```python
from build123d import *

# Parameters (mm, degrees)
SKETCH1_W                       = 44
SKETCH1_H                       = 150
BOSS_EXTRUDE1_DEPTH             = 8
CUT_EXTRUDE3_DEPTH              = 5
SKETCH3_OUTSIDE_W               = 77.304
SKETCH3_OUTSIDE_H               = 183.304
CUT_EXTRUDE4_DEPTH              = 8
CBORE_FOR_M3_SBHCS1_D           = 3.4
CBORE_FOR_M3_SBHCS1_CBORE_D     = 6.7
CBORE_FOR_M3_SBHCS1_CBORE_DEPTH = 1.65


with BuildPart() as part:
    # Sketch1 → Boss-Extrude1 (new body)
    with BuildSketch(Plane(origin=(0, 0, 0), x_dir=(0, 0, -1), z_dir=(1, 0, 0))):
        with Locations((22, 75)):
            Rectangle(SKETCH1_W, SKETCH1_H)
    extrude(amount=BOSS_EXTRUDE1_DEPTH)

    # Sketch2 → Cut-Extrude3 (cut)
    with BuildSketch(Plane(origin=(0, 0, 0), x_dir=(0, 0, -1), z_dir=(1, 0, 0))):
        Polygon((22, 19), (18.535898385, 17), (18.535898385, 13), (22, 11), (25.464101615, 13), (25.464101615, 17), align=None)
    extrude(amount=CUT_EXTRUDE3_DEPTH, mode=Mode.SUBTRACT)

    # Sketch3 outside → Cut-Extrude4 (cut)
    with BuildSketch(Plane(origin=(8, 0, 0), x_dir=(0, 0, -1), z_dir=(1, 0, 0))):
        with Locations((22, 75)):
            Rectangle(SKETCH3_OUTSIDE_W, SKETCH3_OUTSIDE_H)
        with BuildLine():
            Line((11, 150), (11, 28.564659966))
            ThreePointArc((11, 28.564659966), (10.591663047, 25.736232842), (9.4, 23.13879598))
            ThreePointArc((9.4, 23.13879598), (22, 0), (34.6, 23.13879598))
            ThreePointArc((34.6, 23.13879598), (33.408336953, 25.736232842), (33, 28.564659966))
            Line((33, 28.564659966), (33, 150))
            Line((33, 150), (11, 150))
        make_face(mode=Mode.SUBTRACT)
    extrude(amount=-CUT_EXTRUDE4_DEPTH, mode=Mode.SUBTRACT)

    # CBORE for M3 SBHCS1 (through all)
    with Locations(Plane(origin=(8, 0, 0), x_dir=(0, 0, -1), z_dir=(1, 0, 0))):
        with Locations((22, 15)):
            CounterBoreHole(CBORE_FOR_M3_SBHCS1_D / 2, CBORE_FOR_M3_SBHCS1_CBORE_D / 2, CBORE_FOR_M3_SBHCS1_CBORE_DEPTH)


solid = part.part
```
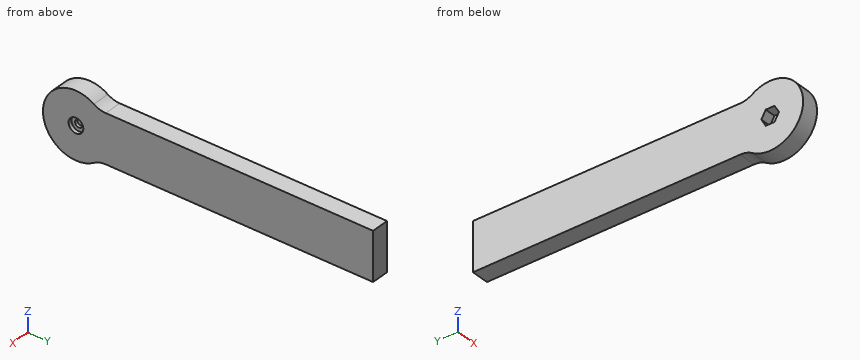
CAD build for the part. Positions are in the model's coordinates, mm. Give positions to 0.01 mm unless a question says otherwise; leave off trailing zeros. Write each loop counter-clockwise with the first axis right and the second up, starting at its lowest first coordinate (ties: lowest second). Pieces come first, ordered by that corner, then holes. Notation, with made-up numbers: M 40,12 L 73,12 A34 ccw 73,43 Z; hole C 60,78 d6. An arc over 180 degrees is marked long. Return JSON: item names as keys, results as strings. Group by question number.
(1) Flat gauge pins, fed straight in: pin 1 Ø1 at (x, y) = (1.5, 108) entering from -Z; pin 2 Ø4 at (x, y) = (5, 122) entering from +Z; pin 3 Ø2 at (y, z) = (14, -22.5) entering from -X. Where does each tip first touch, or does it go through?
(2) Band-saw the part on A-A (y = 15). Give the cut face in (x, z), and give its area (3 significant figures).
(3) Band-saw the part on B-B (x = 1.75). Give the cut face in (y, z), and give its area (3 significant figures).
(4) Band-saw the part on C-C (y = 98). Give the cut face in (x, z), and give its area (3 significant figures).
(5) Band-saw the part on D-D (z = -13.5). Give the cut face in (x, y), and give its area (3 significant figures).
(6) Drill centre lines: L1, parallel to Y at x = 7.05, z = -22; L2, parallel to Y at x = 5.5, z = -22; L3, parallel to Z at x = 4.75, y = 40. Where is each one in solid material? Low to high. Write a range as [from, to].
Entries:
{
 "1": {"pin 1": "stops at z = -33", "pin 2": "stops at z = -11", "pin 3": "stops at x = 5"},
 "2": {"outline": "M 0,-37 L 8,-37 L 8,-25.35 L 6.35,-25.35 L 6.35,-23.7 L 5,-23.7 L 5,-25.46 L 0,-25.46 Z; M 0,-18.54 L 5,-18.54 L 5,-20.3 L 6.35,-20.3 L 6.35,-18.65 L 8,-18.65 L 8,-7 L 0,-7 Z", "area": "190 mm^2"},
 "3": {"outline": "M 23.14,-34.6 A10 cw 28.56,-33 L 150,-33 L 150,-11 L 28.56,-11 A10 cw 23.14,-9.4 A15 ccw long Z; hole M 11,-22 L 13,-25.46 L 17,-25.46 L 19,-22 L 17,-18.54 L 13,-18.54 Z", "area": "3,340 mm^2"},
 "4": {"outline": "M 0,-33 L 8,-33 L 8,-11 L 0,-11 Z", "area": "176 mm^2"},
 "5": {"outline": "M 0,2.64 L 8,2.64 L 8,150 L 0,150 Z", "area": "1,180 mm^2"},
 "6": {"L1": "y = [0, 11.65], [18.35, 150]", "L2": "y = [0, 13.3], [16.7, 150]", "L3": "z = [-33, -11]"}
}
